Work out the finished part from the listing and answer in its coordinate system (mm). A direction names the side the tool comes from. Give positions to 0.01 mm unless a question says otherwise; leave off trailing zeros. Loops run counter-clockwise (first coordinate to the right, second up) from the corner with the lowest first, then second, coordinate; pieces in that order, holes last. Notation, with made-up numbers: (73, 36) - (96, 36) arc R26 ccw to (96, 55) - close; hole circle Ø10 at (-10.75, 37.5). An arc over 180 degrees is marked (long way). One line per question, with ' | ' between items. Start each with the question number.
1. Each of these flat-tipped pins is pushed along its axis until it touches: pin 1 (2 mm diameter, centred on x = 8.66, z = 5, fed in from +Y); pin 2 (10 mm diameter, centred on x = 11, z = -11, fed in from +Y); pin 3 (3 mm diameter, centred on y = 3, z = -15, fed in from -X); pin 4 (1.5 mm diameter, centred on x = -17.5, y = 12, fed in from -Z). Where does it stop, or does it pass through?
2. Which of the six approach directions +Z, -Z, +X, -X, +Y, -Y give full straight-line access (tool end or side, diameter ignored) to faces 4 (the face through (15.25, 13.18, 16.89)), 5 (the face through (-22.697, 10.465, 0.052)), 6 (the face through (14.07, 13.79, -17.89))?
3. Section A-A (z = 0) is taken. Determine the outline of the cut face in (x, y), plus the area to 3 significant figures.
4. For a pull along Z with two mould halves and no side action, classify faces 1 (the face through (-5, 0, 0)), 2 (the face through (-0.7, 1.3, 19)), 3 (the face through (8.46, 13.93, -21.13)) as released by +Z, released by -Z, zero draft, split by the parting line, or undercut.
5. Section C-C (y = 6.5) is taken. Determine the outline of the cut face in (x, z).
6. Section D-D (x = -21) is taken. Determine the outline of the cut face in (y, z), plus the area to 3 significant figures.
7. Find the intervals of material crossed by line 1 (X direction, y = 0.6, z = -10); line 2 (X direction, y = 1.6, z = 5); line 3 (Y direction, x = -4.5, z = 7), in increasing order.
8. Section B-B (y = 16) is taken. Determine the outline of the cut face in (x, z), plus the area to 3 significant figures.
from build123d import *

# Parameters (mm, degrees)
SKETCH1_R             = 23.5
BOSS_EXTRUDE1_DEPTH   = 2.54
F_2_CLEARANCE_HOLE2_D = 2.4384
SKETCH4_R             = 23.5
SKETCH4_R_2           = 22
BOSS_EXTRUDE2_DEPTH   = 16.3576
F_2_CLEARANCE_HOLE1_D = 2.4384
SKETCH7_R             = 1.2192
SKETCH7_R_2           = 0.75
CUT_EXTRUDE1_DEPTH    = 39.2311298
CUT_EXTRUDE2_DEPTH    = 10
CUT_EXTRUDE3_DEPTH    = 10
CUT_EXTRUDE4_DEPTH    = 10


with BuildPart() as part:
    # Sketch1 → Boss-Extrude1 (new body)
    with BuildSketch(Plane(origin=(0, 0, 0), x_dir=(1, 0, 0), z_dir=(0, 1, 0))):
        with Locations(Location((0, 0, 0), (0, 0, 270))):
            Circle(SKETCH1_R)
    extrude(amount=BOSS_EXTRUDE1_DEPTH)

    # #2 Clearance Hole2 (through all)
    with Locations(Plane(origin=(0, 2.54, -10), x_dir=(0, 0, 1), z_dir=(0, 1, 0))):
        with Locations((0, 0), (15, 8.660254038), (15, -8.660254038)):
            Hole(F_2_CLEARANCE_HOLE2_D / 2)

    # Sketch4 → Boss-Extrude2 (add)
    with BuildSketch(Plane(origin=(0, 2.54, 0), x_dir=(1, 0, 0), z_dir=(0, 1, 0))):
        with Locations(Location((0, 0, 0), (0, 0, 270))):
            Circle(SKETCH4_R)
        with Locations(Location((0, 0, 0), (0, 0, 270))):
            Circle(SKETCH4_R_2, mode=Mode.SUBTRACT)
    extrude(amount=BOSS_EXTRUDE2_DEPTH)

    # #2 Clearance Hole1 (through all)
    with Locations(Plane(origin=(0, 0, 20), x_dir=(0, 0, -1), z_dir=(0, -1, 0))):
        with Locations((0, 0), (30, 17.320508076), (30, -17.320508076)):
            Hole(F_2_CLEARANCE_HOLE1_D / 2)

    # Sketch7 → Cut-Extrude1 (cut, through all)
    with BuildSketch(Plane.XZ):
        with Locations(Location((-8, 13.856406461, 0), (0, 0, 270))):
            Circle(SKETCH7_R)
        with Locations(Location((8.0005, 13.857272486, 0), (0, 0, 270))):
            Circle(SKETCH7_R)
        with Locations(Location((16.0015, 0.000866025, 0), (0, 0, 270))):
            Circle(SKETCH7_R)
        with Locations(Location((8.002, -13.856406461, 0), (0, 0, 270))):
            Circle(SKETCH7_R)
        with Locations(Location((-7.9985, -13.857272486, 0), (0, 0, 270))):
            Circle(SKETCH7_R)
        with Locations(Location((-15.9995, -0.000866025, 0), (0, 0, 270))):
            Circle(SKETCH7_R)
        with Locations(Location((0, 0, 0), (0, 0, 270))):
            Circle(SKETCH7_R_2)
    extrude(amount=-CUT_EXTRUDE1_DEPTH, mode=Mode.SUBTRACT)

    # Sketch9 → Cut-Extrude2 (cut)
    with BuildSketch(Plane(origin=(11.75, 0, 20.351596989), x_dir=(0.866025403784438, 0, -0.5000000000000012), z_dir=(0.5000000000000011, 0, 0.8660254037844379))):
        with BuildLine():
            Line((-4.7625, 7.3025), (-4.7625, 18.8976))
            Line((-4.7625, 18.8976), (4.7625, 18.8976))
            Line((4.7625, 18.8976), (4.7625, 7.3025))
            ThreePointArc((4.7625, 7.3025), (0, 2.54), (-4.7625, 7.3025))
        make_face()
    extrude(amount=-CUT_EXTRUDE2_DEPTH, mode=Mode.SUBTRACT)

    # Sketch10 → Cut-Extrude3 (cut)
    with BuildSketch(Plane(origin=(11.75, 0, -20.351596989), x_dir=(-0.8660254037844415, 0, -0.49999999999999517), z_dir=(0.4999999999999951, 0, -0.8660254037844414))):
        with BuildLine():
            Line((-3.2385, 8.8138), (-3.2385, 18.8976))
            Line((-3.2385, 18.8976), (3.2385, 18.8976))
            Line((3.2385, 18.8976), (3.2385, 8.8138))
            ThreePointArc((3.2385, 8.8138), (0, 5.5753), (-3.2385, 8.8138))
        make_face()
    extrude(amount=-CUT_EXTRUDE3_DEPTH, mode=Mode.SUBTRACT)

    # Sketch11 → Cut-Extrude4 (cut)
    with BuildSketch(Plane.ZY.offset(23.5)):
        with BuildLine():
            Line((-2.38125, 12.84605), (-2.38125, 18.8976))
            Line((-2.38125, 18.8976), (2.38125, 18.8976))
            Line((2.38125, 18.8976), (2.38125, 12.84605))
            ThreePointArc((2.38125, 12.84605), (0, 10.4648), (-2.38125, 12.84605))
        make_face()
    extrude(amount=-CUT_EXTRUDE4_DEPTH, mode=Mode.SUBTRACT)


solid = part.part
Conclusion:
1) pin 1: through | pin 2: y = 2.54 | pin 3: x = -19.24 | pin 4: z = -16.48
2) face 4: +Z, +Y | face 5: -X, +Y | face 6: -Z, +Y
3) outline: (-23.5, 0) - (-17.22, 0) - (-17.22, 2.54) - (-22, 2.54) - (-22, 10.46) - (-23.5, 10.46) - close; (-14.78, 0) - (-0.75, 0) - (-0.75, 2.54) - (-14.78, 2.54) - close; (0.75, 0) - (14.78, 0) - (14.78, 2.54) - (0.75, 2.54) - close; (17.22, 0) - (23.5, 0) - (23.5, 18.9) - (22, 18.9) - (22, 2.54) - (17.22, 2.54) - close | area: 140 mm²
4) face 1: zero draft | face 2: undercut | face 3: released by +Z
5) outline: (6.68, 20.96) - (7.45, 22.29) arc R23.5 ccw (long way) to (9.73, -21.39) - (8.98, -20.08) arc R22 cw (long way) to start; (12.9, -17.82) - (13.66, -19.12) arc R23.5 ccw to (15.58, 17.59) - (14.81, 16.27) arc R22 cw to start
6) outline: (0, -10.55) - (18.9, -10.55) - (18.9, -6.56) - (2.54, -6.56) - (2.54, 6.56) - (18.9, 6.56) - (18.9, 10.55) - (0, 10.55) - close | area: 184 mm²
7) line 1: -21.27 to -18.54, -16.1 to -1.22, 1.22 to 16.1, 18.54 to 21.27 | line 2: -22.96 to -9.88, -7.44 to 7.44, 9.88 to 22.96 | line 3: 0 to 2.54
8) outline: (-23.38, -2.38) arc R23.5 ccw to (8.83, -21.78) - (8.08, -20.46) arc R22 cw to (-21.87, -2.38) - close; (-23.38, 2.38) - (-21.87, 2.38) arc R22 cw to (6.61, 20.98) - (7.38, 22.31) arc R23.5 ccw to start; (13.68, -17.23) - (14.44, -18.54) arc R23.5 ccw to (15.63, 17.55) - (14.86, 16.22) arc R22 cw to start | area: 183 mm²
